Geometry check sheet. Reference: the model listing, model coordinates, mm. Face numbers are marked on the shaded views. A direction names the side the tool comes from. Round coordinates to 2 decimals unless told otherwise and drop trailing zeros. Order: outer loops, then holes, each group sorted by start corner. A loop starts at its lowest first (then second) coordinate and runs counter-clockwise, first axis right, second up.
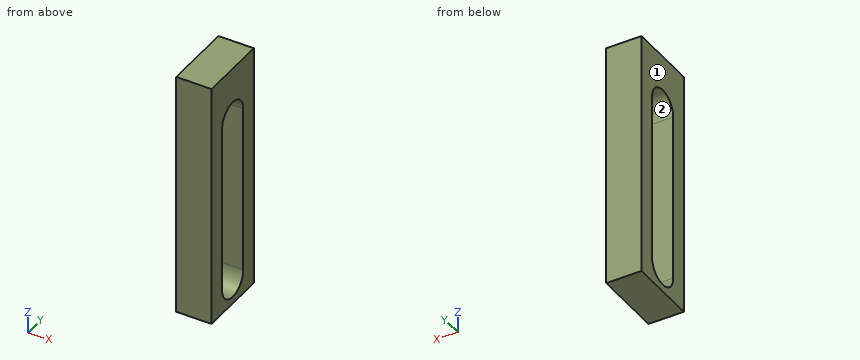
```python
from build123d import *

# Parameters (mm, degrees)
F1_DEPTH = 1.5875
F3_DEPTH = 3.176


with BuildPart() as f1:
    # F0 (on Right) → F1 (new body, symmetric)
    with BuildSketch(Plane.YZ):
        Polygon((-3.175, 0), (0, 0), (3.175, 0), (3.175, 22.225), (-3.175, 22.225), align=None)
    extrude(amount=F1_DEPTH, both=True)

    # F2 (on face) → F3 (cut, through all)
    with BuildSketch(Plane.YZ.offset(1.5875)):
        with BuildLine():
            ThreePointArc((1.5875, 17.4625), (0, 19.05), (-1.5875, 17.4625))
            Line((-1.5875, 17.4625), (-1.5875, 2.2225))
            ThreePointArc((-1.5875, 2.2225), (0, 0.635), (1.5875, 2.2225))
            Line((1.5875, 2.2225), (1.5875, 17.4625))
        make_face()
    extrude(amount=-F3_DEPTH, mode=Mode.SUBTRACT)


solid = f1.part
```
(1) Sectioned sample at A-A, the plane z = 6.25. Record the cut outline in (x, y) (1 decimal), and give its area (3 significant figures).
Returned:
outline: (-1.6, -3.2) - (1.6, -3.2) - (1.6, -1.6) - (-1.6, -1.6) - close; (-1.6, 1.6) - (1.6, 1.6) - (1.6, 3.2) - (-1.6, 3.2) - close
area: 10.1 mm2
(2) Sectioned sample at B-B, the plane x = -0.2. Record the cut outline in (y, z) (1 decimal).
Returned:
outline: (-3.2, 0) - (3.2, 0) - (3.2, 22.2) - (-3.2, 22.2) - close; hole (-1.6, 2.2) arc R1.6 ccw to (1.6, 2.2) - (1.6, 17.5) arc R1.6 ccw to (-1.6, 17.5) - close
(3) Material ranges on line 1 (Y direction, x = 0.3, z = 8.5) (1 decimal); line 2 (Z direction, x = -0.4, y = -1) (3 decimals); line 3 (Z direction, x = -0.2, y = -0.75) (3 decimals), recorded low to high.
Returned:
line 1: y = -3.2 to -1.6, 1.6 to 3.2
line 2: z = 0 to 0.99, 18.695 to 22.225
line 3: z = 0 to 0.823, 18.862 to 22.225
(4) Set-up check for the marked faces 1 and 2: record each of +Z, -Z, +X, -X, +Y, -Y from which the full face is reachable in a straight line by a thin tool's end or side.
Returned:
face 1: +Z, -Z, -X, +Y, -Y
face 2: +X, -X
